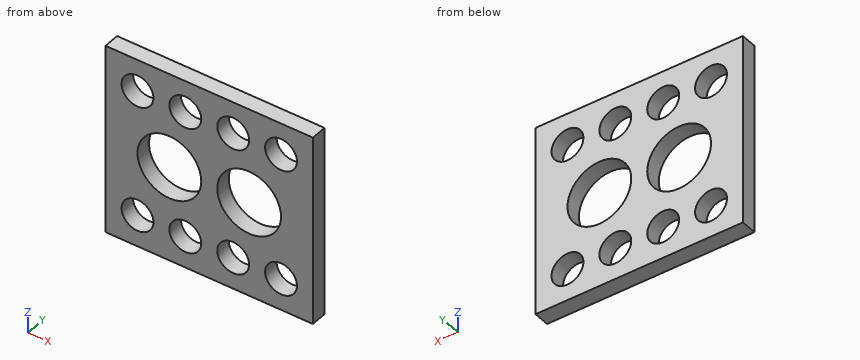
```python
from build123d import *

# Parameters (mm, degrees)
SKETCH1_W           = 165.1
SKETCH1_H           = 152.4
BOSS_EXTRUDE1_DEPTH = 12.7
SKETCH2_R           = 12.7
CUT_EXTRUDE1_DEPTH  = 12.7
SKETCH3_R           = 25.4
CUT_EXTRUDE2_DEPTH  = 12.7


with BuildPart() as part:
    # Sketch1 → Boss-Extrude1 (new body)
    with BuildSketch(Plane(origin=(0, 0, 0), x_dir=(1, 0, 0), z_dir=(0, 1, 0))):
        with Locations((82.55, 76.2)):
            Rectangle(SKETCH1_W, SKETCH1_H)
    extrude(amount=-BOSS_EXTRUDE1_DEPTH)

    # Sketch2 → Cut-Extrude1 (cut)
    with BuildSketch(Plane(origin=(0, 0, 0), x_dir=(1, 0, 0), z_dir=(0, 1, 0))):
        with Locations((25.4, 127)):
            Circle(SKETCH2_R)
        with Locations((63.5, 127)):
            Circle(SKETCH2_R)
        with Locations((101.6, 127)):
            Circle(SKETCH2_R)
        with Locations((139.7, 127)):
            Circle(SKETCH2_R)
        with Locations((63.5, 25.4)):
            Circle(SKETCH2_R)
        with Locations((101.6, 25.4)):
            Circle(SKETCH2_R)
        with Locations((139.7, 25.4)):
            Circle(SKETCH2_R)
        with Locations((25.4, 25.4)):
            Circle(SKETCH2_R)
    extrude(amount=-CUT_EXTRUDE1_DEPTH, mode=Mode.SUBTRACT)

    # Sketch3 → Cut-Extrude2 (cut)
    with BuildSketch(Plane(origin=(0, 0, 0), x_dir=(1, 0, 0), z_dir=(0, 1, 0))):
        with Locations((50.8, 76.2)):
            Circle(SKETCH3_R)
        with Locations((114.3, 76.2)):
            Circle(SKETCH3_R)
    extrude(amount=-CUT_EXTRUDE2_DEPTH, mode=Mode.SUBTRACT)


solid = part.part
```
Can you work these out from the model? Positions are in its coordinate system, mm. Round coordinates to 2 decimals unless told otherwise and drop trailing zeros. Loops run counter-clockwise (first coordinate to the right, second up) from the corner with the lowest first, then second, coordinate; pieces in that order, holes last. Notation, with made-up numbers: (-40, 18.5) -> (6, 18.5) arc R25 ccw to (6, 54.5) -> close; hole circle Ø6 at (11.5, 62.5). An arc over 180 degrees is marked (long way). Answer in a Markdown table with one row per item.
Item 1: If I drill on probe 1 along X at (y, z) = (-5.5, -127); probe 2 along X at (y, z) = (-4, -76.2); probe 3 along Z at (x, y) = (55, -10), over which ranges is the centre line in solid material (lowest first)?
Answer block:
| item | result |
|---|---|
| probe 1 | 0 to 12.7, 38.1 to 50.8, 76.2 to 88.9, 114.3 to 127, 152.4 to 165.1 |
| probe 2 | 0 to 25.4, 76.2 to 88.9, 139.7 to 165.1 |
| probe 3 | -152.4 to -136.44, -117.56 to -101.25, -51.15 to -34.84, -15.96 to 0 |
Item 2: Suppose I cut it at A-A, the plane z = -25.4. List the corners of the cut face in (x, y) for me, plus the area to 3 significant figures.
Answer block:
| item | result |
|---|---|
| outline | (0, -12.7) -> (12.7, -12.7) -> (12.7, 0) -> (0, 0) -> close; (38.1, -12.7) -> (50.8, -12.7) -> (50.8, 0) -> (38.1, 0) -> close; (76.2, -12.7) -> (88.9, -12.7) -> (88.9, 0) -> (76.2, 0) -> close; (114.3, -12.7) -> (127, -12.7) -> (127, 0) -> (114.3, 0) -> close; (152.4, -12.7) -> (165.1, -12.7) -> (165.1, 0) -> (152.4, 0) -> close |
| area | 806 mm² |
Item 3: Suppose I cut it at D-D, the plane y = -6.5. Give the number of separate pieces and of enclosed holes in the cut face, plus the area to 3 significant figures.
Answer block:
| item | result |
|---|---|
| separate pieces | 1 |
| enclosed holes | 10 |
| area | 17,100 mm² |
Item 4: Suppose I cut it at C-C, the plane z = -76.2. List the corners of the cut face in (x, y) for me.
Answer block:
| item | result |
|---|---|
| outline | (0, -12.7) -> (25.4, -12.7) -> (25.4, 0) -> (0, 0) -> close; (76.2, -12.7) -> (88.9, -12.7) -> (88.9, 0) -> (76.2, 0) -> close; (139.7, -12.7) -> (165.1, -12.7) -> (165.1, 0) -> (139.7, 0) -> close |
Item 5: Suppose I cut it at B-B, the plane x = 101.6. List the corners of the cut face in (y, z) for me, plus the area to 3 significant figures.
Answer block:
| item | result |
|---|---|
| outline | (-12.7, -152.4) -> (0, -152.4) -> (0, -139.7) -> (-12.7, -139.7) -> close; (-12.7, -114.3) -> (0, -114.3) -> (0, -98.2) -> (-12.7, -98.2) -> close; (-12.7, -54.2) -> (0, -54.2) -> (0, -38.1) -> (-12.7, -38.1) -> close; (-12.7, -12.7) -> (0, -12.7) -> (0, 0) -> (-12.7, 0) -> close |
| area | 732 mm² |
